Input: part model. Units: mm. Frame: model coordinates. Face numbers are marked on the shaded views. A direction names the side the tool comes from. Round coordinates to 2 decimals unless told otherwise and drop trailing zeros. Order: outer loops, then holes, each group sorted by start corner. A loop starts at its lowest first (then second) coordinate and runs counter-clockwise, first axis right, second up.
Item 1: Mould query, pull axis Y, two halves, no side actions, for the marked faces 6, 7 and 8. Classes: released by +Y, released by -Y, zero draft, split by the parting line, or undercut.
Item 2: Line query: L1, parallel to X at y = 8.5, z = 0.5; L2, parallel to Y at x = -68, z = -16; L3, parallel to Z at x = -53, y = 16. Output: solid intervals per line, ascending.
Item 3: Cut plane A-A on x = -68.5. Output: boundary loops of the cut face in (y, z).
Item 4: Cut plane D-D on z = 14. Output: boundary loops of the cut face in (x, y), then the cut area to 3 significant figures.
Item 5: Cut plane C-C on z = 0. Output: boundary loops of the cut face in (x, y).
Item 6: First-contact query: pin 1 (10 mm diameter, centred on y = 23, z = -16.5, fed in from +X); pin 2 (18 mm diameter, centred on x = -68.5, y = 38, fed in from -Z); pin 3 (5 mm diameter, centred on y = 8.5, z = -3, fed in from +X); pin 4 (10 mm diameter, centred on y = 10, z = 6.5, fed in from +X). Flat tips, straight axial feed; report the tip coordinate or a pass-through.
Item 7: Reachability of the marked faces 1, 2, 3, 4 and 5 from +Z, -Z, +X, -X, +Y, -Y: full face, straight path, thin tool, end or side. Return the list, or none.
Item 8: Cut plane B-B on y = 16.5. Output: boundary loops of the cut face in (x, z), then the cut area to 3 significant figures.
```python
from build123d import *

# Parameters (mm, degrees)
BOSS_EXTRUDE1_DEPTH = 9
SKETCH4_R           = 7
BOSS_EXTRUDE2_DEPTH = 9


with BuildPart() as part:
    # Sketch2 → Boss-Extrude1 (new body)
    with BuildSketch(Plane(origin=(0, 0, 0), x_dir=(1, 0, 0), z_dir=(0, 1, 0))):
        with BuildLine():
            Line((0, -20), (-86, -20))
            Line((-86, -20), (-86, 20))
            Line((-86, 20), (0, 20))
            ThreePointArc((0, 20), (20, 0), (0, -20))
        make_face()
        with BuildLine():
            Line((-24, 7), (0, 7))
            ThreePointArc((0, 7), (7, 0), (0, -7))
            Line((0, -7), (-24, -7))
            ThreePointArc((-24, -7), (-31, 0), (-24, 7))
        make_face(mode=Mode.SUBTRACT)
    extrude(amount=BOSS_EXTRUDE1_DEPTH)

    # Sketch4 → Boss-Extrude2 (add)
    with BuildSketch(Plane.XY.offset(20)):
        with BuildLine():
            Line((-86, 0), (-86, 38))
            ThreePointArc((-86, 38), (-68.5, 55.5), (-51, 38))
            Line((-51, 38), (-51, 0))
            Line((-51, 0), (-86, 0))
        make_face()
        with Locations((-68.5, 38)):
            Circle(SKETCH4_R, mode=Mode.SUBTRACT)
    boss_extrude2 = extrude(amount=-BOSS_EXTRUDE2_DEPTH)

    # Mirror1: Boss-Extrude2 across plane
    add(boss_extrude2.mirror(Plane.XY))


solid = part.part
```
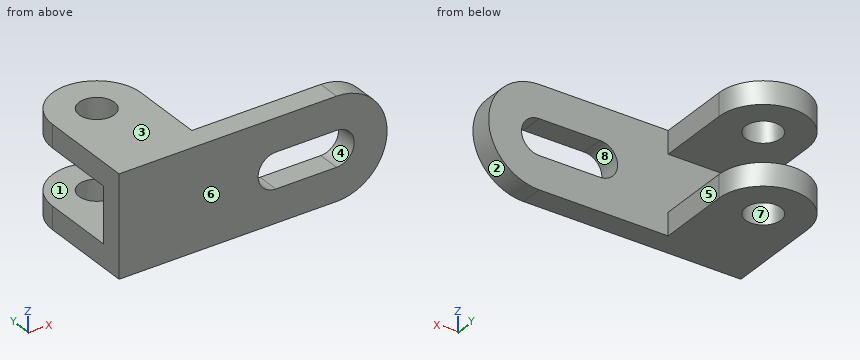
From the geometry:
1. face 6: released by -Y
1. face 7: undercut
1. face 8: zero draft
2. L1: x = -86 to -30.98, 6.98 to 19.99
2. L2: y = 0 to 31.02, 44.98 to 55.49
2. L3: z = -20 to -11, 11 to 20
3. outline: (0, -20) - (31, -20) - (31, -11) - (9, -11) - (9, 11) - (31, 11) - (31, 20) - (0, 20) - close; (45, -20) - (55.5, -20) - (55.5, -11) - (45, -11) - close; (45, 11) - (55.5, 11) - (55.5, 20) - (45, 20) - close
4. outline: (-86, 0) - (14.28, 0) - (14.28, 9) - (-51, 9) - (-51, 38) arc R17.5 ccw to (-86, 38) - close; hole circle Ø14 at (-68.5, 38)
4. area: 2,240 mm2
5. outline: (-86, 0) - (-31, 0) - (-31, 9) - (-86, 9) - close; (7, 0) - (20, 0) - (20, 9) - (7, 9) - close
6. pin 1: stops at x = -51
6. pin 2: stops at z = -20
6. pin 3: stops at x = 19.99
6. pin 4: stops at x = 19.94
7. face 1: +X, -X, +Y
7. face 2: +X, +Y, -Y
7. face 3: +Z, +X, -X, +Y, -Y
7. face 4: +Y, -Y
7. face 5: +Z, -Z, +X, +Y
8. outline: (-86, -20) - (-51, -20) - (-51, -11) - (-86, -11) - close; (-86, 11) - (-51, 11) - (-51, 20) - (-86, 20) - close
8. area: 630 mm2
